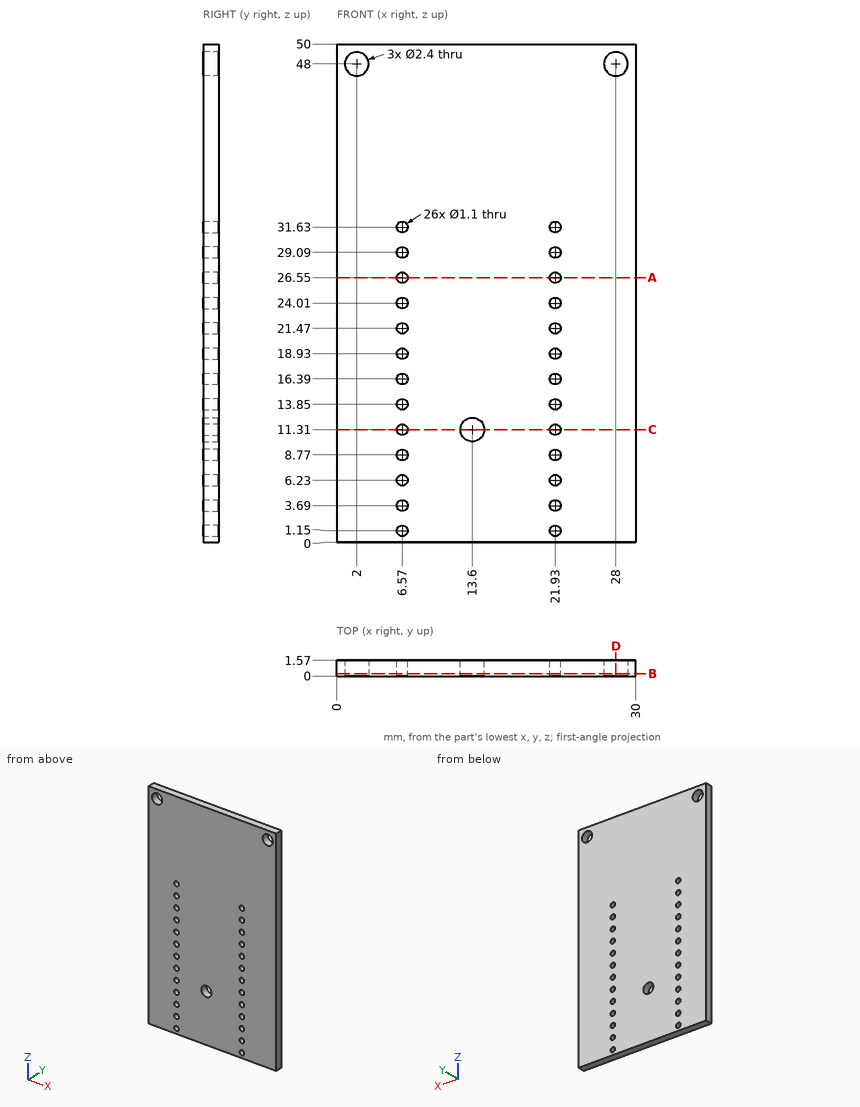
Could you check a few things on this drawing? It's one solid part, dimensions in mm from its lowest x, y, z. Coordinates: 2 decimals unless noted, no trailing zeros. Write each loop counter-clockwise with the first axis right and the second up, starting at its lowest first coordinate (ties: lowest second). Pieces come first, ordered by that corner, then holes. Notation, with made-up numbers: (86.25, 49.25) - (133.25, 49.25) arc R27 ccw to (133.25, 70.25) - close; hole circle Ø6 at (25, -9.5). An arc over 180 degrees is marked (long way). Write item = value, one per line.
1) Please list where these lines run through material, in increasing order: line 1 (X direction, y = 0.8, z = 13.85); line 2 (X direction, y = 0.45, z = 6); line 3 (Z direction, x = 13, y = 0.5). Write a range as [from, to].
Result set:
line_1 = [0, 6.02], [7.12, 21.38], [22.48, 30]
line_2 = [0, 6.07], [7.07, 21.43], [22.43, 30]
line_3 = [0, 10.27], [12.35, 50]
2) Suppose I cut it at C-C on z = 11.31. Please give me the cut outline in (x, y).
Result set:
outline = (0, 0) - (6.02, 0) - (6.02, 1.57) - (0, 1.57) - close; (7.12, 0) - (12.4, 0) - (12.4, 1.57) - (7.12, 1.57) - close; (14.8, 0) - (21.38, 0) - (21.38, 1.57) - (14.8, 1.57) - close; (22.48, 0) - (30, 0) - (30, 1.57) - (22.48, 1.57) - close
3) Suppose I cut it at A-A on z = 26.55. Please give me the cut outline in (x, y), plus the area to 3 significant figures.
Result set:
outline = (0, 0) - (6.02, 0) - (6.02, 1.57) - (0, 1.57) - close; (7.12, 0) - (21.38, 0) - (21.38, 1.57) - (7.12, 1.57) - close; (22.48, 0) - (30, 0) - (30, 1.57) - (22.48, 1.57) - close
area = 43.6 mm2
4) Suppose I cut it at B-B on y = 0.25. State how many separate pieces and enclosed holes the cut face has, plus the area to 3 significant figures.
Result set:
separate_pieces = 1
enclosed_holes = 29
area = 1,460 mm2
5) Suppose I cut it at D-D on x = 28. Please give me the cut outline in (y, z).
Result set:
outline = (0, 0) - (1.57, 0) - (1.57, 46.8) - (0, 46.8) - close; (0, 49.2) - (1.57, 49.2) - (1.57, 50) - (0, 50) - close
